Here's how the part is built. I have some questions about the finished solid (model axes, mm). Round coordinates to 2 decimals unless told otherwise and drop trailing zeros. Write each loop counter-clockwise with the first axis right and the second up, starting at its lowest first coordinate (ties: lowest second). Pieces come first, ordered by that corner, then holes. Notation, with made-up numbers: (-24, 46) -> (1, 46) arc R17 cw to (1, 79) -> close; hole circle Ø10 at (74.5, 23). An arc over 180 degrees is marked (long way). Put each result on its own line as item: value. Start each with the question number.
1. We'd pull the mould along X, two halves only. Please class faces 1 (the face through (-36.76, 93.237, 1.61)), 2 (the face through (-13.83, -12.65, 1.57)), 3 (the face through (-13.41, 195.69, 1.57)), 4 (the face through (-12.236, 258.276, 1.61)): +X half, -X half, draft (parallel to the pull), parting line (faces both ways), or undercut.
2. Suppose I cut it at B-B (z = 0.7). Count the separate pieces of the cut face and the enclosed holes in it, then the cut area to 3 significant figures.
3. Suppose I cut it at C-C (y = 238.5). Please give me the cut outline in (x, z) (3 decimals).
4. I need wall thicknesses on probe 1 along X at (y, z) = (66.5, 3.05); probe 2 along X at (y, z) = (88, 0.25); probe 3 along X at (y, z) = (81.5, 0.8). Which ranges of each line are inside material? Lowest first, please. Write a range as from..to.
5. Suppose I cut it at A-A (x = -10). Please give me the cut outline in (y, z) (3 decimals).
Autodesk Inventor part; units mm, degrees
ref_plane "YZ Plane" through (0, 0, 0) normal (1, 0, 0) x (0, 1, 0)
ref_plane "XZ Plane" through (0, 0, 0) normal (0, 1, 0) x (-1, 0, 0)
ref_plane "XY Plane" through (0, 0, 0) normal (0, 0, 1) x (1, 0, 0)
sketch "Sketch1" plane through (0, 0, 0) normal (0, 0, 1) x (1, 0, 0)
  line L0 (0, 0) -> (-24.739, 111.5906)
  line L1 (0, 0) -> (114.3, 0) construction
  line L2 (-24.739, 111.5906) -> (0, 223.1813)
  line L3 (0, 223.1813) -> (-25.4, 223.1813)
  line L4 (-24.739, 111.5906) -> (-50.139, 111.5906)
  line L5 (0, 0) -> (-25.4, 0)
  line L6 (-25.4, 0) -> (-50.139, 111.5906)
  line L7 (-25.4, 223.1813) -> (-50.139, 111.5906)
  arc A0 (0, 223.1813) -> (-25.4, 223.1813) centre (-12.7, 223.1813) ccw
  arc A1 (-25.4, 0) -> (0, 0) centre (-12.7, 0) ccw
  circle A2 centre (-12.7, 0) radius 6.35
  circle A3 centre (-12.7, 223.1813) radius 6.35
  line L8 (0, 0) -> (-28.396, 128.086)
  line L9 (-28.396, 128.086) -> (1.8406, 264.4745)
  line L10 (-28.396, 128.086) -> (111.304, 128.086) construction
  line L11 (1.8406, 264.4745) -> (-23.5594, 264.4745)
  line L12 (-28.396, 128.086) -> (-53.796, 128.086)
  line L13 (-53.796, 128.086) -> (-23.5594, 264.4745)
  line L14 (0, 0) -> (-25.4, 0)
  line L15 (-53.796, 128.086) -> (-25.4, 0)
  arc A4 (-25.4, 0) -> (0, 0) centre (-12.7, 0) ccw
  circle A5 centre (-12.7, 0) radius 6.35
  arc A6 (1.8406, 264.4745) -> (-23.5594, 264.4745) centre (-10.8594, 264.4745) ccw
  circle A7 centre (-10.8594, 264.4745) radius 6.35
  dimension "d0" = 114.3
  dimension "d1" = 102.5
  dimension "d2" = 114.3
  dimension "d3" = 155
  dimension "d4" = 25.4
  dimension "d5" = 25.4
  dimension "d6" = 25.4
  dimension "d7" = 12.7
  dimension "d8" = 12.7
  dimension "d9" = 12.7
  dimension "d10" = 12.7
  dimension "d24" = 139.7
  dimension "d25" = 77.5
  dimension "d26" = 25.4
  dimension "d27" = 25.4
  dimension "d28" = 12.7
  dimension "d29" = 12.7
extrude "Extrusion3" add sketch "Sketch1" along normal blind 6.35 contours L5 A2 L6 L4 L0 | A1 L5 A2 | L4 L7 L12 L8 | L15 L12 L7 | L12 L7 L3 A3 L9 | L9 A3 L3 A0 | A0 L7 L12 L13 L11 A7 L9 | A3 L3 L9 | L3 A3 L9 | L11 A7 A6 picked at (-23.0997, 224.6964) picked at (-15.0808, 222.6929) picked at (-15.082, 223.6647)
sketch "Sketch3" plane through (0, 0, 6.35) normal (0, 0, 1) x (1, 0, 0)
  line L0 (1.8406, 264.4745) -> (-28.396, 128.086)
  line L1 (-53.796, 128.086) -> (-23.5594, 264.4745)
  line L2 (-28.396, 128.086) -> (-53.796, 128.086)
  line L3 (-28.396, 128.086) -> (-23.8337, 107.5068)
  line L4 (-28.396, 128.086) -> (0, 0)
  line L5 (-25.4, 0) -> (-53.796, 128.086)
  line L6 (-41.096, 128.086) -> (-36.3335, 103.1365)
  circle A0 centre (-10.8594, 264.4745) radius 6.35
  line L7 (-41.096, 128.086) -> (-33.9522, 90.6617)
  line L8 (-41.096, 128.086) -> (-39.9054, 121.8486)
  line L9 (-41.096, 128.086) -> (-28.396, 128.086)
  line L10 (-41.096, 128.086) -> (-33.9522, 90.6617)
  line L11 (-33.9522, 90.6617) -> (-28.8722, 90.6617) construction
  circle A1 centre (-33.9522, 90.6617) radius 3.81
  line L12 (-38.6033, 115.0277) -> (-36.8935, 106.0705)
  line L13 (-35.4604, 115.6269) -> (-24.0304, 115.6269) construction
  circle A2 centre (-33.3166, 104.3997) radius 1.27
  dimension "d42" = 25.4
  dimension "d50" = 38.1
  dimension "d51" = 6.35
  dimension "d59" = 7.62
  dimension "d82" = 2.54
sketch "Sketch5" plane through (0, 0, 6.35) normal (0, 0, 1) x (1, 0, 0)
  circle A0 centre (-10.8594, 264.4745) radius 7.4295
  circle A1 centre (-12.7, 0) radius 7.4295
  point P0 (0, 0)
  dimension "d76" = 14.859
  dimension "d77" = 14.859
extrude "Extrusion14" cut sketch "Sketch5" against normal blind 25.4
extrude "Extrusion15" cut sketch "Sketch3" against normal blind 25.4 contours A1 | A2
sketch "Sketch6" plane through (0, 0, 6.35) normal (0, 0, 1) x (1, 0, 0)
  circle A0 centre (-33.3166, 104.3997) radius 1.27
  line L0 (0, 0) -> (-28.396, 128.086)
  line L1 (-33.3166, 104.3997) -> (-7.9166, 104.3997) construction
  line L2 (-33.3166, 104.3997) -> (-27.8191, 79.6018)
  line L3 (-33.3166, 104.3997) -> (-7.9166, 104.3997) construction
  line L4 (-27.8191, 79.6018) -> (-25.0703, 67.2029)
  line L5 (-25.0703, 67.2029) -> (-22.3215, 54.8039)
  line L6 (-22.3215, 54.8039) -> (-19.5727, 42.4049)
  line L7 (-19.5727, 42.4049) -> (-16.8239, 30.006)
  circle A1 centre (-27.8191, 79.6018) radius 1.27
  circle A2 centre (-25.0703, 67.2029) radius 1.27
  circle A3 centre (-22.3215, 54.8039) radius 1.27
  circle A4 centre (-19.5727, 42.4049) radius 1.27
  circle A5 centre (-16.8239, 30.006) radius 1.27
  dimension "d89" = 25.4
  dimension "d90" = 77.5
  dimension "d91" = 12.7
  dimension "d92" = 12.7
  dimension "d93" = 12.7
  dimension "d94" = 12.7
  dimension "d95" = 2.54
  dimension "d96" = 2.54
  dimension "d97" = 2.54
  dimension "d98" = 2.54
  dimension "d99" = 2.54
extrude "Extrusion16" cut sketch "Sketch6" against normal blind 25.4 contours A5 | A4 L7 L6 | L6 L7 A4 | A3 L6 L5 | L5 L6 A3 | A2 L5 L4 | L4 L5 A2 | A1 L4 L2 | L2 L4 A1
sketch "Sketch7" plane through (0, 0, 6.35) normal (0, 0, 1) x (1, 0, 0)
  circle A0 centre (-33.3166, 104.3997) radius 1.27
  line L0 (-33.3166, 104.3997) -> (-36.559, 119.2908)
  circle A1 centre (-36.559, 119.2908) radius 1.27
  point P0 (0, 0)
  dimension "d102" = 15.24
  dimension "d103" = 2.54
extrude "Extrusion17" cut sketch "Sketch7" against normal blind 25.4 contours A1
sketch "Sketch8" plane through (0, 0, 6.35) normal (0, 0, 1) x (1, 0, 0)
  circle A0 centre (-36.559, 119.2908) radius 1.27
  circle A1 centre (-22.3215, 54.8039) radius 1.27
  circle A2 centre (-19.5727, 42.4049) radius 1.27
  circle A3 centre (-25.0703, 67.2029) radius 1.27
  circle A4 centre (-16.8239, 30.006) radius 1.27
  circle A5 centre (-27.8191, 79.6018) radius 1.27
  circle A6 centre (-33.9522, 90.6617) radius 3.81
  circle A7 centre (-33.3166, 104.3997) radius 1.27
  circle A8 centre (-10.8594, 264.4745) radius 7.4295
  circle A9 centre (-12.7, 0) radius 7.4295
  arc A10 (-25.4, 0) -> (0, 0) centre (-12.7, 0) ccw
  line L0 (-28.396, 128.086) -> (0, 0)
  line L1 (1.8406, 264.4745) -> (-28.396, 128.086)
  arc A11 (1.8406, 264.4745) -> (-23.5594, 264.4745) centre (-10.8594, 264.4745) ccw
  line L2 (-53.796, 128.086) -> (-23.5594, 264.4745)
  line L3 (-25.4, 0) -> (-53.796, 128.086)
extrude "Extrusion18" cut sketch "Sketch8" against normal blind 3.175
sketch "Sketch9" plane through (0, 0, 3.175) normal (0, 0, 1) x (1, 0, 0)
  circle A0 centre (-36.559, 119.2908) radius 1.27
  line L0 (-36.559, 119.2908) -> (-28.396, 169.4307)
  line L1 (-36.559, 119.2908) -> (-44.179, 119.2908)
  circle A1 centre (-33.3166, 104.3997) radius 1.27
  line L2 (-33.3166, 104.3997) -> (-40.9366, 104.3997)
  circle A2 centre (-27.8191, 79.6018) radius 1.27
  line L3 (-27.8191, 79.6018) -> (-35.4391, 79.6018)
  circle A3 centre (-25.0703, 67.2029) radius 1.27
  line L4 (-25.0703, 67.2029) -> (-32.6903, 67.2029)
  circle A4 centre (-22.3215, 54.8039) radius 1.27
  line L5 (-22.3215, 54.8039) -> (-29.9415, 54.8039)
  circle A5 centre (-19.5727, 42.4049) radius 1.27
  line L6 (-19.5727, 42.4049) -> (-27.1927, 42.4049)
  circle A6 centre (-16.8239, 30.006) radius 1.27
  line L7 (-16.8239, 30.006) -> (-24.4439, 30.006)
  circle A7 centre (-27.1927, 42.4049) radius 1.27
  circle A8 centre (-24.4439, 30.006) radius 1.27
  circle A9 centre (-29.9415, 54.8039) radius 1.27
  circle A10 centre (-32.6903, 67.2029) radius 1.27
  circle A11 centre (-35.4391, 79.6018) radius 1.27
  circle A12 centre (-40.9366, 104.3997) radius 1.27
  circle A13 centre (-44.179, 119.2908) radius 1.27
  line L8 (-36.559, 119.2908) -> (-34.5183, 131.8258)
  line L9 (-34.5183, 131.8258) -> (-32.4775, 144.3607)
  line L10 (-32.4775, 144.3607) -> (-30.4367, 156.8957)
  line L11 (-28.396, 169.4307) -> (-25.6472, 181.8296)
  line L12 (-28.396, 169.4307) -> (-15.696, 169.4307) construction
  line L13 (-25.6472, 181.8296) -> (-22.8984, 194.2286)
  line L14 (-22.8984, 194.2286) -> (-20.1496, 206.6275)
  line L15 (-20.1496, 206.6275) -> (-27.7696, 206.6275)
  line L16 (-22.8984, 194.2286) -> (-30.5184, 194.2286)
  line L17 (-25.6472, 181.8296) -> (-33.2672, 181.8296)
  line L18 (-28.396, 169.4307) -> (-36.016, 169.4307)
  line L19 (-30.4367, 156.8957) -> (-38.0567, 156.8957)
  line L20 (-32.4775, 144.3607) -> (-40.0975, 144.3607)
  line L21 (-34.5183, 131.8258) -> (-42.1383, 131.8258)
  circle A14 centre (-27.7696, 206.6275) radius 1.27
  circle A15 centre (-20.1496, 206.6275) radius 1.27
  circle A16 centre (-30.5184, 194.2286) radius 1.27
  circle A17 centre (-22.8984, 194.2286) radius 1.27
  circle A18 centre (-33.2672, 181.8296) radius 1.27
  circle A19 centre (-25.6472, 181.8296) radius 1.27
  circle A20 centre (-36.016, 169.4307) radius 1.27
  circle A21 centre (-28.396, 169.4307) radius 1.27
  circle A22 centre (-42.1383, 131.8258) radius 1.27
  circle A23 centre (-40.0975, 144.3607) radius 1.27
  circle A24 centre (-38.0567, 156.8957) radius 1.27
  circle A25 centre (-34.5183, 131.8258) radius 1.27
  circle A26 centre (-32.4775, 144.3607) radius 1.27
  circle A27 centre (-30.4367, 156.8957) radius 1.27
  point P0 (0, 0)
  dimension "d108" = 50.8
  dimension "d109" = 7.62
  dimension "d110" = 7.62
  dimension "d111" = 7.62
  dimension "d112" = 7.62
  dimension "d113" = 7.62
  dimension "d114" = 7.62
  dimension "d115" = 7.62
  dimension "d116" = 2.54
  dimension "d117" = 2.54
  dimension "d118" = 2.54
  dimension "d119" = 2.54
  dimension "d120" = 2.54
  dimension "d121" = 2.54
  dimension "d122" = 2.54
  dimension "d123" = 12.7
  dimension "d124" = 12.7
  dimension "d125" = 12.7
  dimension "d126" = 12.7
  dimension "d127" = 77.5
  dimension "d128" = 12.7
  dimension "d129" = 12.7
  dimension "d130" = 7.62
  dimension "d131" = 7.62
  dimension "d132" = 7.62
  dimension "d133" = 7.62
  dimension "d134" = 7.62
  dimension "d135" = 7.62
  dimension "d136" = 7.62
  dimension "d137" = 2.54
  dimension "d138" = 2.54
  dimension "d139" = 2.54
  dimension "d140" = 2.54
  dimension "d141" = 2.54
  dimension "d142" = 2.54
  dimension "d143" = 2.54
  dimension "d144" = 2.54
  dimension "d145" = 2.54
  dimension "d146" = 2.54
  dimension "d147" = 2.54
  dimension "d148" = 2.54
  dimension "d149" = 2.54
  dimension "d150" = 2.54
extrude "Extrusion19" cut sketch "Sketch9" against normal blind 3.175 contours A13 | A22 | A23 | A24 | A20 | A18 | A16 | A14 | A15 L15 L14 | L14 L15 A15 | A17 L16 L13 | L13 L14 A17 | A19 L17 L11 | L11 L13 A19 | A21 L18 L0 | L0 L11 A21 | A27 L19 L0 | L0 A27 | A26 L20 L0 | L0 A26 | A25 L21 L0 | L0 A25 | L21 A25 L0 | L20 A26 L0 | L19 A27 L0 | L18 A21 L11 | L17 A19 L13 | L16 A17 L14 | A12 | A11 | A10 | A9 | A7 | A8
sketch "Sketch10" plane through (0, 0, 3.175) normal (0, 0, 1) x (1, 0, 0)
  circle A0 centre (-33.3166, 104.3997) radius 1.27
  circle A1 centre (-33.3166, 104.3997) radius 1.27
  circle A2 centre (-40.9366, 104.3997) radius 1.27
  circle A3 centre (-40.9366, 104.3997) radius 1.27
  point P0 (0, 0)
extrude "Extrusion20" add sketch "Sketch10" against normal blind 3.175
sketch "Sketch11" plane through (0, 0, 3.175) normal (0, 0, 1) x (1, 0, 0)
  point P0 (0, 0)
sketch "Sketch12" plane through (0, 0, 3.175) normal (0, 0, 1) x (1, 0, 0)
  point P0 (0, 0)
fillet "Fillet1" radius 10.16 6 edges at (-25.4, 0, 1.5875) (0, 0, 1.5875) (-53.796, 128.086, 1.5875) (-28.396, 128.086, 1.5875) (1.8406, 264.4745, 1.5875) (-23.5594, 264.4745, 1.5875)
sketch "Sketch13" plane through (0, 0, 3.175) normal (0, 0, 1) x (1, 0, 0)
  point P0 (0, 0)
sketch "Sketch14" plane through (0, 0, 3.175) normal (0, 0, 1) x (1, 0, 0)
  circle A0 centre (-12.7, 0) radius 7.4295
  circle A1 centre (-12.7, 0) radius 6.35
  circle A2 centre (-10.8594, 264.4745) radius 7.4295
  circle A3 centre (-10.8594, 264.4745) radius 6.35
  circle A4 centre (-10.8594, 264.4745) radius 7.4295
  point P0 (0, 0)
  dimension "d156" = 12.7
  dimension "d157" = 12.7
extrude "Extrusion21" add sketch "Sketch14" against normal blind 3.175
properties part number "angle v3 inside"
Verdict:
1. face 1: undercut
1. face 2: parting line
1. face 3: +X half
1. face 4: undercut
2. separate pieces: 1
2. enclosed holes: 29
2. area: 6,790 mm^2
3. outline: (-29.318, 0) -> (-3.918, 0) -> (-3.918, 3.175) -> (-29.318, 3.175) -> close
4. probe 1: x = -40.14..-33.75, -31.63..-26.13, -24.01..-14.74
4. probe 2: x = -44.91..-36.68, -31.23..-19.51
4. probe 3: x = -43.47..-18.07
5. outline: (-12.41, 0) -> (-5.747, 0) -> (-5.747, 3.175) -> (-12.41, 3.175) -> close; (5.747, 0) -> (45.107, 0) -> (45.107, 3.175) -> (5.747, 3.175) -> close; (211.065, 0) -> (258.183, 0) -> (258.183, 3.175) -> (211.065, 3.175) -> close; (270.766, 0) -> (277.145, 0) -> (277.145, 3.175) -> (270.766, 3.175) -> close
